```python
from build123d import *

# Parameters (mm, degrees)
SKETCH1_W           = 3
SKETCH1_H           = 44.45
BOSS_EXTRUDE1_DEPTH = 25.4
SKETCH10_R          = 1.5
CUT_EXTRUDE1_DEPTH  = 125.927823604


with BuildPart() as part:
    # Sketch1 → Boss-Extrude1 (new body)
    with BuildSketch(Plane(origin=(0, 0, 0), x_dir=(1, 0, 0), z_dir=(0, 1, 0))):
        with Locations((-13.038815819, 45.598435945)):
            Rectangle(SKETCH1_W, SKETCH1_H)
        Polygon((25.128862589, 23.373435945), (29.128862589, 23.373435945), (29.128862589, 71.823435945), (25.128862589, 71.823435945), (25.128862589, 67.823435945), align=None)
        Polygon((-67.439681, 71.812406658), (-63.450710286, 67.823435945), (-14.538815819, 67.823435945), (-11.538815819, 67.823435945), (25.128862589, 67.823435945), (25.128862589, 71.823435945), (-69.857244767, 71.823435945), (-69.857244767, 69.394842891), align=None)
        Polygon((-69.857244767, 68.573116176), (-69.107564536, 67.823435945), (-63.450710286, 67.823435945), (-67.439681, 71.812406658), (-69.857244767, 69.394842891), align=None)
        Polygon((-69.857244767, 67.823435945), (-69.107564536, 67.823435945), (-69.857244767, 68.573116176), align=None)
        Polygon((-69.107564536, 67.823435945), (-21.829137411, 20.54500882), (-21.829137411, 23.373435945), (-19.000710286, 23.373435945), (-63.450710286, 67.823435945), align=None)
        Polygon((-21.829137411, 20.54500882), (-21.829137411, -28.584564055), (-15.829137411, -28.584564055), (-15.829137411, -25.584564055), (-18.829137411, -25.584564055), (-18.829137411, 19.373435945), (26.128862589, 19.373435945), (26.128862589, -25.584564055), (23.128862589, -25.584564055), (23.128862589, -28.584564055), (29.128862589, -28.584564055), (29.128862589, 23.373435945), (25.128862589, 23.373435945), (-11.538815819, 23.373435945), (-14.538815819, 23.373435945), (-19.000710286, 23.373435945), align=None)
        Polygon((-21.829137411, 23.373435945), (-21.829137411, 20.54500882), (-19.000710286, 23.373435945), align=None)
    extrude(amount=BOSS_EXTRUDE1_DEPTH)

    # Sketch10 → Cut-Extrude1 (cut, through all)
    with BuildSketch(Plane(origin=(0, 0, -71.823435945), x_dir=(-1, 0, 0), z_dir=(0, 0, -1))):
        with Locations((39.857244767, 6.7)):
            Circle(SKETCH10_R)
        with Locations((39.857244767, 18.7)):
            Circle(SKETCH10_R)
        with Locations((-9.128862589, 6.7)):
            Circle(SKETCH10_R)
        with Locations((-9.128862589, 18.7)):
            Circle(SKETCH10_R)
    extrude(amount=-CUT_EXTRUDE1_DEPTH, mode=Mode.SUBTRACT)


solid = part.part
```
Here's how the part is built. I have some questions about the finished solid (model axes, mm). A direction names the side the tool comes from. Coordinates: 2 decimals unless noted, no trailing zeros. Order: outer loops, then holes, each group sorted by start corner. A loop starts at its lowest first (then second) coordinate and runs counter-clockwise, first axis right, second up. Notation, with made-up numbers: (-2, -26.5) - (38, -26.5) arc R21 ccw to (38, -12.5) - close; hole circle Ø11 at (62.25, -17.5). An arc over 180 degrees is marked (long way). One line per question, with ' | ' between items. Start each with the question number.
1. If we section it at C-C (x = -50): Write out the boundary of the cut face in (y, z).
2. I'm going to push flat-ended pins straight in: pin 1 Ø4 at (x, y) = (9.13, 6.7) entering from +Z; pin 2 Ø5 at (x, y) = (-39.86, 6.7) entering from +Z; pin 3 Ø12.5 at (y, z) = (14, -35.5) entering from -X; pin 4 Ø2.5 at (x, y) = (9.13, 18.7) entering from +Z. Where does each tip first touch, or does it pass through?
3. If we section it at D-D (z = -48.5): Write out the boundary of the cut face in (x, y), and give its area (3 significant figures).
4. If we section it at A-A (y = 3): Write out the boundary of the cut face in (x, z) (3 decimals).
5. If we section it at B-B (z = 7.5): Write out the boundary of the cut face in (x, y), and give its area (3 significant figures).
6. Please list where these lines run through material, in increasing order: line 1 along Z through (x, y) = (-17.5, 17); line 2 along X through (y, z) = (4, -1); line 3 along Z through (x, y) = (20.5, 3.5). Write a range as [from, to].
7. Which directions (+Z, -Z, +X, -X, +Y, -Y) give clear straight access to the entire face, cutting with the end or side of a thin tool? Please do faces 1 (the flat face through (25, 13, 25.585)), 2 (the cylindrical face through (-38.36, 18.77, -69.85)), 3 (the flat face through (-21.829, 13, 4)).
8. If we mould it in two halves opening along Z, with no side actions, what happens to faces 4 (the flat face through (25.129, 13, -46)), 5 (the flat face through (-15.829, 13, 27)), 6 (the flat face through (-45.799, 12.522, -44.515))? For each: released by +Z, released by -Z, zero draft, split by the parting line, or undercut.
Model answer:
1) outline: (0, -71.82) - (25.4, -71.82) - (25.4, -67.82) - (0, -67.82) - close; (0, -54.37) - (25.4, -54.37) - (25.4, -48.72) - (0, -48.72) - close
2) pin 1: stops at z = -19.37 | pin 2: stops at z = -36.08 | pin 3: stops at x = -43.03 | pin 4: passes through
3) outline: (-49.78, 0) - (-44.13, 0) - (-44.13, 25.4) - (-49.78, 25.4) - close; (-14.54, 0) - (-11.54, 0) - (-11.54, 25.4) - (-14.54, 25.4) - close; (25.13, 0) - (29.13, 0) - (29.13, 25.4) - (25.13, 25.4) - close | area: 321 mm²
4) outline: (-69.857, -71.823) - (29.129, -71.823) - (29.129, 28.585) - (23.129, 28.585) - (23.129, 25.585) - (26.129, 25.585) - (26.129, -19.373) - (-18.829, -19.373) - (-18.829, 25.585) - (-15.829, 25.585) - (-15.829, 28.585) - (-21.829, 28.585) - (-21.829, -20.545) - (-69.108, -67.823) - (-69.857, -67.823) - close; hole (-63.451, -67.823) - (-14.539, -67.823) - (-14.539, -23.373) - (-19.001, -23.373) - close; hole (-11.539, -67.823) - (25.129, -67.823) - (25.129, -23.373) - (-11.539, -23.373) - close
5) outline: (-21.83, 0) - (-18.83, 0) - (-18.83, 25.4) - (-21.83, 25.4) - close; (26.13, 0) - (29.13, 0) - (29.13, 25.4) - (26.13, 25.4) - close | area: 152 mm²
6) line 1: z = [-71.82, -67.82], [-23.37, -19.37], [25.58, 28.58] | line 2: x = [-21.83, -18.83], [26.13, 29.13] | line 3: z = [-71.82, -67.82], [-23.37, -19.37]
7) face 1: +Y, -Y | face 2: +Z, -Z | face 3: +Z, -X, +Y, -Y
8) face 4: undercut | face 5: zero draft | face 6: released by +Z
